Autodesk Inventor part; units mm, degrees
ref_plane "YZ Plane" through (0, 0, 0) normal (1, 0, 0) x (0, 1, 0)
ref_plane "XZ Plane" through (0, 0, 0) normal (0, 1, 0) x (-1, 0, 0)
ref_plane "XY Plane" through (0, 0, 0) normal (0, 0, 1) x (1, 0, 0)
sketch "Sketch1" plane through (0, 0, 0) normal (0, 1, 0) x (-1, 0, 0)
  line L0 (46.6892, 43.4449) -> (-45.937, 43.4449)
  line L1 (-45.937, 43.4449) -> (-45.937, -47.0251)
  line L2 (-45.937, -47.0251) -> (46.6892, -47.0251)
  line L3 (46.6892, -47.0251) -> (46.6892, 43.4449)
  point P0 (0, 0)
extrude "Extrusion1" add sketch "Sketch1" along normal blind 12.7
sketch "Sketch2" plane through (0, 12.7, 0) normal (0, 1, 0) x (1, 0, 0)
  line L0 (-4.6344, -12.9521) -> (-6.35, -0.0003)
  line L1 (-4.6344, -12.9521) -> (0.0041, -12.9521)
  line L2 (0.0041, -12.9521) -> (4.5761, -12.9521)
  line L3 (4.5761, -12.9521) -> (6.35, -0.0003)
  arc A0 (0.004, -17.2664) -> (4.5761, -12.9521) centre (-0.3869, -12.2723) ccw
  arc A1 (-4.6344, -12.9521) -> (0.004, -17.2664) centre (0.1159, -12.4955) ccw
  line L4 (-4.6401, 12.8677) -> (0.0124, 12.8677)
  line L5 (0.0124, 12.8677) -> (4.5844, 12.8677)
  arc A2 (0.0041, 17.2458) -> (-4.6401, 12.8677) centre (0.1159, 12.4749) ccw
  arc A3 (4.5844, 12.8677) -> (0.0041, 17.2458) centre (-0.3881, 12.2505) ccw
  line L6 (4.5844, 12.8677) -> (6.35, -0.0003)
  line L7 (-4.6401, 12.8677) -> (-6.35, -0.0003)
  line L8 (-6.35, -0.0003) -> (-12.7, -0.0003)
  line L9 (6.35, -0.0003) -> (12.7, -0.0003)
  arc A4 (-12.7, -0.0003) -> (-12.0319, -1.6197) centre (-10.414, -0.0048) ccw
  line L10 (-6.35, -2.0323) -> (-12.0319, -1.6197)
  line L11 (-6.35, 2.0317) -> (-12.0319, 1.6102)
  arc A5 (-12.0319, 1.6102) -> (-12.7, -0.0092) centre (-10.414, -0.0048) ccw
  line L12 (-6.35, -2.0323) -> (-6.0808, -2.0323)
  line L13 (-6.35, 2.0317) -> (-6.08, 2.0317)
  line L14 (6.35, -0.0003) -> (12.7, -0.0003)
  arc A6 (12.7, -0.0003) -> (12.0319, 1.6191) centre (10.414, 0.0041) ccw
  line L15 (6.35, 2.0317) -> (12.0319, 1.6191)
  line L16 (6.35, -2.0323) -> (12.0319, -1.6108)
  arc A7 (12.0319, -1.6108) -> (12.7, 0.0085) centre (10.414, 0.0041) ccw
  line L17 (6.35, -2.0323) -> (6.0717, -2.0323)
  line L18 (6.35, 2.0317) -> (6.0712, 2.0317)
  point P0 (0, 0)
  point P1 (0.6686, -44.2967)
  point P2 (0.0037, 25.7566)
  point P3 (-0.0257, 7.5764)
  point P4 (0.0037, -0.0211)
  point P5 (12.0319, 1.6191)
  dimension "d12" = 4.572
  dimension "d16" = 4.572
  dimension "d20" = 2.032
  dimension "d21" = 2.032
  dimension "d22" = 2.286
  dimension "d25" = 2.032
extrude "Extrusion2" cut sketch "Sketch2" against normal blind 5.08
sketch "Sketch3" plane through (0, 12.7, 0) normal (0, 1, 0) x (1, 0, 0)
  circle A0 centre (0, 0) radius 7.112
  dimension "d30" = 14.224
extrude "Extrusion3" cut sketch "Sketch3" against normal blind 7.62
Can you work these out from the model? Positions are in its coordinate system, mm. A direction names the side the tool comes from. Round coordinates to 2 decimals unless told otherwise and drop trailing zeros. Write each loop counter-clockwise with the first axis right and the second up, starting at its lowest first coordinate (ties: lowest second). Pieces come first, ordered by that corner, then holes. Notation, with made-up numbers: (53.5, -12.5) - (78.5, -12.5) arc R18 ccw to (78.5, 7.5) - close; hole circle Ø2 at (14, 33.25). An arc over 180 degrees is marked (long way). Write each question's results on one line, items separated by ' | '. Start each with the question number.
1) Suppose I cut it at A-A (y = 10.5). List the corners of the cut face in (x, z) for me, and give its area (3 significant figures).
2) Which directions (+Z, -Z, +X, -X, +Y, -Y) give clear straight access to the entire face, cutting with the end or side of a thin tool? Please do faces 4 (the flat face through (45.937, 6, -1)), 5 (the flat face through (-10, 7.62, 0)).
3) Suppose I cut it at C-C (z = -11). List the corners of the cut face in (x, y) for me, and give its area (3 significant figures).
4) Suppose I cut it at B-B (z = 10.5). List the corners of the cut face in (x, y) for me, and give its area (3 significant figures).
5) For pin 1 Ø3 at (x, z) = (10, 0.5) entering from +Y; pin 2 Ø3.5 at (x, z) = (1, 11.5) entering from +Y, each with a flat end and sliding along its axis, tell me the tip position at first contact or that it passes through.
6) We'd pull the mould along Z, two halves only. Please class faces 1 (the flat face through (0, 0, -1)), 2 (the flat face through (-1, 6, 43.445)), 3 (the flat face through (5.175, 10.196, -8.566)): released by +Z, released by -Z, zero draft, split by the parting line, or undercut.
7) Please list where these lines run through material, in increasing order: line 1 (Z direction, x = 0, y = 10.25); line 2 (X direction, y = 7.5, z = 0); line 3 (X direction, y = 10, z = 0).
Here are the results:
1) outline: (-46.69, -47.03) - (45.94, -47.03) - (45.94, 43.44) - (-46.69, 43.44) - close; hole (-12.7, 0) arc R2.29 ccw to (-12.03, -1.61) - (-6.83, -2) arc R7.11 ccw to (-5.8, -4.11) - (-4.64, -12.87) arc R4.77 ccw to (0, -17.25) arc R5.01 ccw to (4.58, -12.87) - (5.78, -4.14) arc R7.11 ccw to (6.83, -2) - (12.03, -1.62) arc R2.29 ccw to (12.7, 0) arc R2.29 ccw to (12.03, 1.61) - (6.83, 2) arc R7.11 ccw to (5.78, 4.14) - (4.58, 12.95) arc R5.01 ccw to (0, 17.27) arc R4.77 ccw to (-4.63, 12.95) - (-5.81, 4.11) arc R7.11 ccw to (-6.83, 2) - (-12.03, 1.62) arc R2.29 ccw to start | area: 7,990 mm2
2) face 4: +Z, -Z, +X, +Y, -Y | face 5: +Y
3) outline: (-46.69, 0) - (45.94, 0) - (45.94, 12.7) - (4.84, 12.7) - (4.84, 7.62) - (-4.89, 7.62) - (-4.89, 12.7) - (-46.69, 12.7) - close | area: 1,130 mm2
4) outline: (-46.69, 0) - (45.94, 0) - (45.94, 12.7) - (4.91, 12.7) - (4.91, 7.62) - (-4.96, 7.62) - (-4.96, 12.7) - (-46.69, 12.7) - close | area: 1,130 mm2
5) pin 1: stops at y = 12.7 | pin 2: stops at y = 7.62
6) face 1: zero draft | face 2: released by +Z | face 3: undercut
7) line 1: z = -47.03 to -17.25, 17.27 to 43.44 | line 2: x = -46.69 to -7.11, 7.11 to 45.94 | line 3: x = -46.69 to -12.7, 12.7 to 45.94
